Could you check a few things on this drawing? It's one solid part, dimensions in mm from its lowest x, y, z. A direction names the side the tool comes from. Give positions to 0.01 mm unless a question says otherwise; leave off trailing zeros. Loops run counter-clockwise (first coordinate to the right, second up) from the corner with the lowest first, then second, coordinate; pieces in that order, holes last. Notation, with made-up numbers: (80, 13) - (87, 13) arc R27 cw to (87, 33) - close; hole circle Ø5 at (-30.75, 73.5). An arc over 180 degrees is marked (long way). Write each question's results on one line, items separated by ' | '. Start each with the question number.
(1) Suppose I cut it at C-C (y = 9.5). Please give me the cut outline in (x, z).
(2) Suppose I cut it at A-A (z = 3.75). Please give me the cut outline in (x, y).
(3) Suppose I cut it at D-D (x = 32.5). Please give me the cut outline in (y, z), and give its area (4 significant figures).
(4) If we mould it in two halves opening along X, with no side actions, what happens to the marked faces 6, 7 and 8? For each: released by +X, released by -X, zero draft, split by the parting line, or undercut.
(5) Suppose I cut it at B-B (x = 13). Please give me the cut outline in (y, z), and give its area (3 significant figures).
(6) On a 3-axis mill with a long thin cutter (end or side, diameter ignored), from which of +Z, -Z, +X, -X, +Y, -Y can I reach the whole of each face in a straight line? I mean the marked faces 1, 2, 3, 4 and 5. Say none if no direction works.
(7) For pin 1 (2 mm diameter, centred on x = 23.5, z = 1.5, fed in from +Y); pin 2 (3 mm diameter, centred on x = 22, y = 12, fed in from -Z); pin 3 (2 mm diameter, centred on y = 10, z = 1, fed in from -X), each with a flat end and sliding along its axis, tell me the tip position at first contact or that it passes through.
(8) I need wall thicknesses on line 1 (Y direction, x = 30.5, z = 1); line 2 (Y direction, x = 34, z = 5.5); line 3 (Y direction, x = 11, z = 5.5). Which ranges of each line are inside material? Lowest first, please.
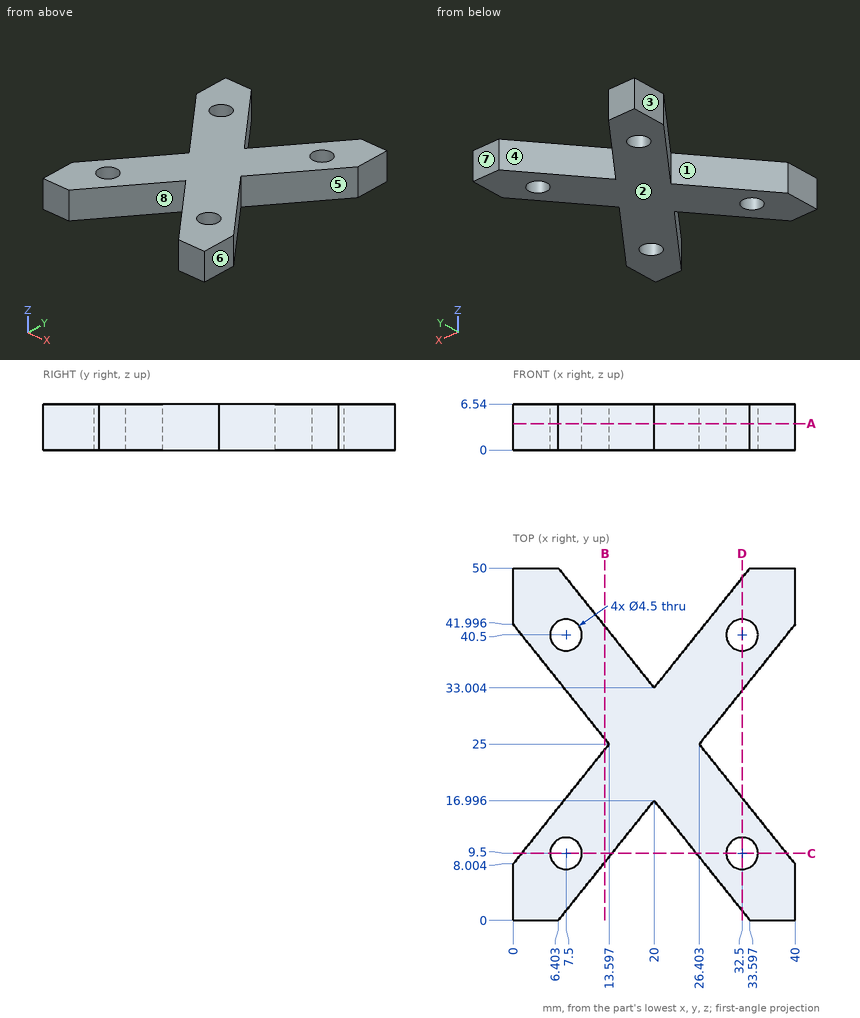
Output values:
1) outline: (1.2, 0) - (5.25, 0) - (5.25, 6.54) - (1.2, 6.54) - close; (9.75, 0) - (14, 0) - (14, 6.54) - (9.75, 6.54) - close; (26, 0) - (30.25, 0) - (30.25, 6.54) - (26, 6.54) - close; (34.75, 0) - (38.8, 0) - (38.8, 6.54) - (34.75, 6.54) - close
2) outline: (0, 0) - (6.4, 0) - (20, 17) - (33.6, 0) - (40, 0) - (40, 8) - (26.4, 25) - (40, 42) - (40, 50) - (33.6, 50) - (20, 33) - (6.4, 50) - (0, 50) - (0, 42) - (13.6, 25) - (0, 8) - close; hole circle Ø4.5 at (7.5, 9.5); hole circle Ø4.5 at (7.5, 40.5); hole circle Ø4.5 at (32.5, 9.5); hole circle Ø4.5 at (32.5, 40.5)
3) outline: (1.37, 0) - (7.25, 0) - (7.25, 6.54) - (1.37, 6.54) - close; (11.75, 0) - (17.38, 0) - (17.38, 6.54) - (11.75, 6.54) - close; (32.62, 0) - (38.25, 0) - (38.25, 6.54) - (32.62, 6.54) - close; (42.75, 0) - (48.63, 0) - (48.63, 6.54) - (42.75, 6.54) - close | area: 150.5 mm2
4) face 6: released by +X | face 7: zero draft | face 8: undercut
5) outline: (8.25, 0) - (24.25, 0) - (24.25, 6.54) - (8.25, 6.54) - close; (25.75, 0) - (41.75, 0) - (41.75, 6.54) - (25.75, 6.54) - close | area: 209 mm2
6) face 1: +Z, -Z, -X | face 2: -Z, +X, -X, +Y, -Y | face 3: +Z, -Z, -X, +Y, -Y | face 4: +Z, -Z, +Y | face 5: +Z, -Z, +X
7) pin 1: y = 38.63 | pin 2: through | pin 3: x = 0.8
8) line 1: 3.87 to 8.47, 10.53 to 19.88, 30.12 to 39.47, 41.53 to 46.13 | line 2: 0 to 7.82, 11.18 to 15.5, 34.5 to 38.82, 42.18 to 50 | line 3: 5.75 to 21.75, 28.25 to 44.25
